Verification items for the finished model (mm, model axes). Coordinates: 2 decimals unless noted, no trailing zeros. Write each loop counter-clockwise with the first axis right and the second up, starting at its lowest first coordinate (ties: lowest second). Pieces come first, ordered by that corner, then holes. Notation, with made-up numbers: M 60.25,-15.75 L 99.25,-15.75 A16 ccw 99.25,-8.75 Z; hole C 42.25,-16.75 d10. An arc over 180 degrees is marked long. Answer in a Markdown table with one row per item.
from build123d import *

# Parameters (mm, degrees)
SKETCH1_W           = 381
SKETCH1_H           = 12.7
BOSS_EXTRUDE1_DEPTH = 6.35
SKETCH2_W           = 25.4
SKETCH2_H           = 6.35
CUT_EXTRUDE1_DEPTH  = 7.35
LPATTERN1_COUNT     = 4
LPATTERN1_PITCH     = 95.25


with BuildPart() as part:
    # Sketch1 → Boss-Extrude1 (new body)
    with BuildSketch(Plane(origin=(0, 0, 0), x_dir=(1, 0, 0), z_dir=(0, 1, 0))):
        Rectangle(SKETCH1_W, SKETCH1_H)
    extrude(amount=BOSS_EXTRUDE1_DEPTH)

    # Sketch2 → Cut-Extrude1 (cut, through all)
    with BuildSketch(Plane(origin=(0, 6.35, 0), x_dir=(1, 0, 0), z_dir=(0, 1, 0))):
        with Locations((-142.875, 0)):
            Rectangle(SKETCH2_W, SKETCH2_H)
    cut_extrude1 = extrude(amount=-CUT_EXTRUDE1_DEPTH, mode=Mode.SUBTRACT)

    # LPattern1: Cut-Extrude1 ×4
    with Locations(*[(i * LPATTERN1_PITCH, 0, 0) for i in range(1, LPATTERN1_COUNT)]):
        add(cut_extrude1, mode=Mode.SUBTRACT)


solid = part.part
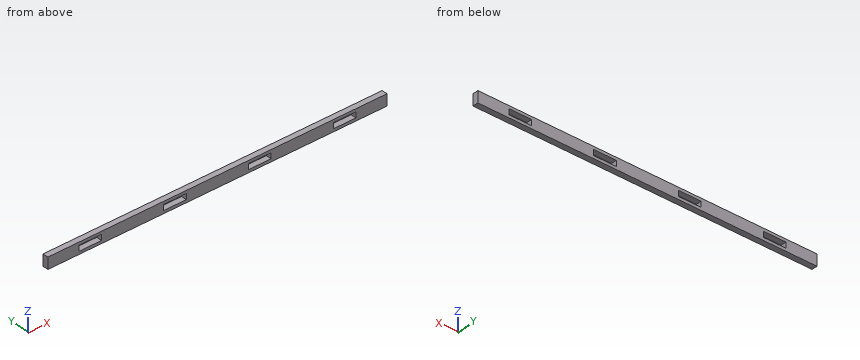
1) Sectioned sample at A-A (x = -56.5). Record the cut outline in (y, z) (3 decimals).
Response values:
| item | result |
|---|---|
| outline | M 0,-6.35 L 6.35,-6.35 L 6.35,-3.175 L 0,-3.175 Z; M 0,3.175 L 6.35,3.175 L 6.35,6.35 L 0,6.35 Z |
2) Sectioned sample at B-B (z = 0.25). Record the cut outline in (x, y) (3 decimals), then the cut area to 3 significant figures.
Response values:
| item | result |
|---|---|
| outline | M -190.5,0 L -155.575,0 L -155.575,6.35 L -190.5,6.35 Z; M -130.175,0 L -60.325,0 L -60.325,6.35 L -130.175,6.35 Z; M -34.925,0 L 34.925,0 L 34.925,6.35 L -34.925,6.35 Z; M 60.325,0 L 130.175,0 L 130.175,6.35 L 60.325,6.35 Z; M 155.575,0 L 190.5,0 L 190.5,6.35 L 155.575,6.35 Z |
| area | 1,770 mm² |
3) Sectioned sample at C-C (y = 5.25). Record the cut outline in (x, z) (3 decimals), then the cut area to 3 significant figures.
Response values:
| item | result |
|---|---|
| outline | M -190.5,-6.35 L 190.5,-6.35 L 190.5,6.35 L -190.5,6.35 Z; hole M -155.575,-3.175 L -130.175,-3.175 L -130.175,3.175 L -155.575,3.175 Z; hole M -60.325,-3.175 L -34.925,-3.175 L -34.925,3.175 L -60.325,3.175 Z; hole M 34.925,-3.175 L 60.325,-3.175 L 60.325,3.175 L 34.925,3.175 Z; hole M 130.175,-3.175 L 155.575,-3.175 L 155.575,3.175 L 130.175,3.175 Z |
| area | 4,190 mm² |
4) Thickness scan on L1, parallel to X at y = 4.5, z = 0.5 (3 decimals); L2, parallel to Z at x = 143, y = 3.5 (3 decimals). Record the ranges inside material, lowest first. Write a range as [from, to].
Response values:
| item | result |
|---|---|
| L1 | x = [-190.5, -155.575], [-130.175, -60.325], [-34.925, 34.925], [60.325, 130.175], [155.575, 190.5] |
| L2 | z = [-6.35, -3.175], [3.175, 6.35] |
